The model under review builds one solid part; all positions refer to its coordinate system, in mm. Face numbers are marked on the shaded views. A direction names the side the tool comes from. Give positions to 0.01 mm unless a question says otherwise; leave off trailing zeros. Order: outer loops, then holes, each group sorted by start corner. A loop starts at its lowest first (then second) coordinate and runs counter-clockwise, first axis right, second up. Notation, with made-up numbers: (52, -18.5) - (68, -18.5) arc R21 ccw to (68, 0.5) - close; hole circle Ø7 at (36.25, 32). An arc over 180 degrees is marked (long way). Write item = value, one per line. Start each with the question number.
1. Machinability: for the marked faces 1 and 2, which of the approach directions +Z, -Z, +X, -X, +Y, -Y give a long, thin tool a straight path to every point of the face, cutting with its end or side? Answer none if there is none.
2. For P1, Ø5, axis at x = 26.5, z = 27, coming from the -Y side, flat-tipped, find the tip position at first contact; note if it passes through.
3. Mouldability with a two-part tool opening along Z and no side actions: class the marked faces 3, 4 and 5 as pulls with the +Z half, pulls with the -Z half, needs draft (parallel to the pull), parting line crosses it, or undercut.
4. We need section A-A, the plane x = -0.5. Give the boundary of the cut face in (y, z).
5. Wall thickness on probe 1 along Z at (x, y) = (13, 8); probe 2 along X at (y, z) = (5.25, 35); probe 3 along Y at (x, z) = (-39, -2.5): over which ranges is each line inside the solid? List them lowest first.
6. We need section C-C, the plane z = -22.5. Give the boundary of the cut face in (x, y), and give its area (3 significant figures).
7. We need section B-B, the plane y = 6. Give the boundary of the cut face in (x, z), and give its area (3 significant figures).
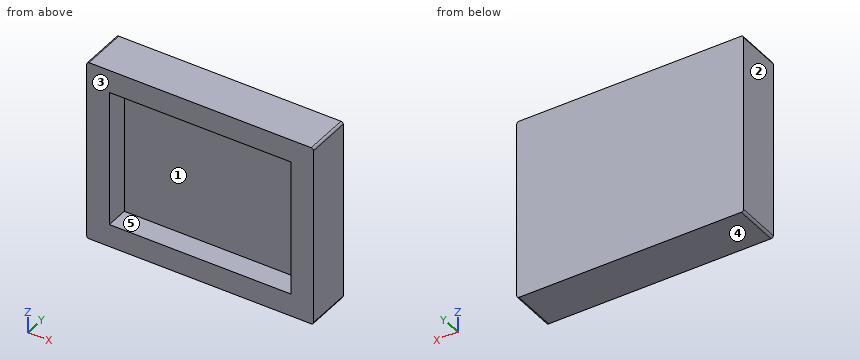
from build123d import *

# Parameters (mm, degrees)
F0_W     = 127
F0_H     = 101.6
F0_W_2   = 101.6
F0_H_2   = 76.2
F1_DEPTH = 25.4
F2_DEPTH = 12.7
F3_R     = 1.27


with BuildPart() as f1:
    # F0 (on Front) → F1 (new body)
    with BuildSketch(Plane.XZ):
        Rectangle(F0_W, F0_H)
        Rectangle(F0_W_2, F0_H_2, mode=Mode.SUBTRACT)
        Rectangle(F0_W_2, F0_H_2)
    extrude(amount=-F1_DEPTH)

    # F0 (on Front) → F2 (cut)
    with BuildSketch(Plane.XZ):
        Rectangle(F0_W_2, F0_H_2)
    extrude(amount=-F2_DEPTH, mode=Mode.SUBTRACT)

    # F3
    f3_edges = [f1.edges().sort_by_distance(p)[0] for p in [
        (-63.5, 12.7, 50.8),
        (63.5, 12.7, 50.8),
        (63.5, 12.7, -50.8),
        (-63.5, 12.7, -50.8),
    ]]
    fillet(f3_edges, radius=F3_R)


solid = f1.part
Model answer:
q1.face_1 = -Y
q1.face_2 = +Z, -Z, -X, +Y, -Y
q2.P1 = 12.7
q3.face_3 = needs draft
q3.face_4 = pulls with the -Z half
q3.face_5 = undercut
q4.outline = (0, -50.8) - (25.4, -50.8) - (25.4, 50.8) - (0, 50.8) - (0, 38.1) - (12.7, 38.1) - (12.7, -38.1) - (0, -38.1) - close
q5.probe_1 = -50.8 to -38.1, 38.1 to 50.8
q5.probe_2 = -63.5 to -50.8, 50.8 to 63.5
q5.probe_3 = 12.7 to 25.4
q6.outline = (-63.5, 0) - (-50.8, 0) - (-50.8, 12.7) - (50.8, 12.7) - (50.8, 0) - (63.5, 0) - (63.5, 25.4) - (-63.5, 25.4) - close
q6.area = 1,940 mm2
q7.outline = (-63.5, -49.53) arc R1.27 ccw to (-62.23, -50.8) - (62.23, -50.8) arc R1.27 ccw to (63.5, -49.53) - (63.5, 49.53) arc R1.27 ccw to (62.23, 50.8) - (-62.23, 50.8) arc R1.27 ccw to (-63.5, 49.53) - close; hole (-50.8, -38.1) - (50.8, -38.1) - (50.8, 38.1) - (-50.8, 38.1) - close
q7.area = 5,160 mm2
